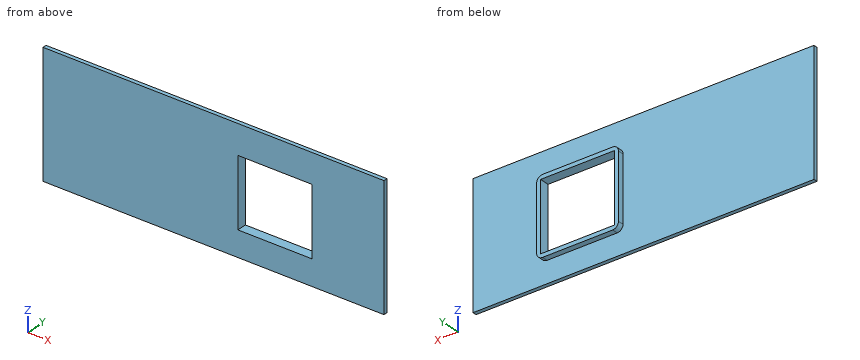
from build123d import *

# Parameters (mm, degrees)
SKETCH1_W           = 42
SKETCH1_H           = 39
SKETCH1_W_2         = 38
SKETCH1_H_2         = 35
BOSS_EXTRUDE1_DEPTH = 3
FILLET2_R           = 3
SKETCH5_W           = 175
SKETCH5_H           = 63
SKETCH5_W_2         = 38
SKETCH5_H_2         = 35
BOSS_EXTRUDE2_DEPTH = 2


with BuildPart() as part:
    # Sketch1 → Boss-Extrude1 (new body)
    with BuildSketch(Plane(origin=(0, 0, 0), x_dir=(1, 0, 0), z_dir=(0, 1, 0))):
        with Locations((-18.389520702, 9.684818057)):
            Rectangle(SKETCH1_W, SKETCH1_H)
        with Locations((-18.389520702, 9.684818057)):
            Rectangle(SKETCH1_W_2, SKETCH1_H_2, mode=Mode.SUBTRACT)
    extrude(amount=BOSS_EXTRUDE1_DEPTH)

    # Fillet2
    fillet2_edges = [part.edges().sort_by_distance(p)[0] for p in [
        (-39.389520702, 1.5, -29.184818057),
        (2.610479298, 1.5, -29.184818057),
        (2.610479298, 1.5, 9.815181943),
        (-39.389520702, 1.5, 9.815181943),
    ]]
    fillet(fillet2_edges, radius=FILLET2_R)

    # Sketch5 → Boss-Extrude2 (add)
    with BuildSketch(Plane.XZ):
        with Locations((-49.889520702, -8.684818057)):
            Rectangle(SKETCH5_W, SKETCH5_H)
        with Locations((-18.389520702, -9.684818057)):
            Rectangle(SKETCH5_W_2, SKETCH5_H_2, mode=Mode.SUBTRACT)
    extrude(amount=BOSS_EXTRUDE2_DEPTH)


solid = part.part
Build history of the part. All positions in model axes, mm. Give positions to 0.01 mm unless a question says otherwise; leave off trailing zeros. Order: outer loops, then holes, each group sorted by start corner. A loop starts at its lowest first (then second) coordinate and runs counter-clockwise, first axis right, second up. Notation, with made-up numbers: M 37,-19 L 75,-19 A23 cw 75,15 Z; hole C -16.75,-6.75 d2. An arc over 180 degrees is marked long. Put each result on its own line as item: value.
Item 1: Slice it at C-C, the plane x = -8. Write the cut outline in (y, z).
From the geometry:
outline: M -2,-40.18 L 0,-40.18 L 0,-29.18 L 3,-29.18 L 3,-27.18 L -2,-27.18 Z; M -2,7.82 L 3,7.82 L 3,9.82 L 0,9.82 L 0,22.82 L -2,22.82 Z
Item 2: Slice it at B-B, the plane y = 1.3. Write the cut outline in (x, z), plus the area to 3 significant figures.
From the geometry:
outline: M -39.39,-26.18 A3 ccw -36.39,-29.18 L -0.39,-29.18 A3 ccw 2.61,-26.18 L 2.61,6.82 A3 ccw -0.39,9.82 L -36.39,9.82 A3 ccw -39.39,6.82 Z; hole M -37.39,-27.18 L 0.61,-27.18 L 0.61,7.82 L -37.39,7.82 Z
area: 300 mm2
Item 3: Probe line 1 (Z direction, x = -22.5, y = -0.45); line 2 (X direction, y = 1.4, z = -8); line 3 (X direction, y = -0.9, z = -24). List the from-to ranges inside material, lowest first. Write a range as [from, to].
From the geometry:
line 1: z = [-40.18, -27.18], [7.82, 22.82]
line 2: x = [-39.39, -37.39], [0.61, 2.61]
line 3: x = [-137.39, -37.39], [0.61, 37.61]
Item 4: Slice it at A-A, the plane z = -9. Write the cut outline in (x, y).
From the geometry:
outline: M -137.39,-2 L -37.39,-2 L -37.39,3 L -39.39,3 L -39.39,0 L -137.39,0 Z; M 0.61,-2 L 37.61,-2 L 37.61,0 L 2.61,0 L 2.61,3 L 0.61,3 Z
Item 5: Slice it at D-D, the plane x = -108. Write the cut outline in (y, z), plus the area to 3 significant figures.
From the geometry:
outline: M -2,-40.18 L 0,-40.18 L 0,22.82 L -2,22.82 Z
area: 126 mm2
Item 6: Flat gauge pins, fed straight in: pin 1 Ø1.5 at (y, z) = (1.5, -3) entering from -X; pin 2 Ø1.5 at (y, z) = (1.5, -2.5) entering from +X; pin 3 Ø0.9 at (x, y) = (-13.5, 1.5) entering from +Z; pin 4 Ø5 at (x, z) = (-2, -14) entering from +Y. Where does each tip first touch, or does it go through?
From the geometry:
pin 1: stops at x = -39.39
pin 2: stops at x = 2.61
pin 3: stops at z = 9.82
pin 4: passes through
